Can you work these out from the model? Positions are in its coordinate system, mm. A direction names the side the tool comes from. Coordinates: 2 decimals unless noted, no trailing zeros. Order: outer loops, then holes, each group sorted by start corner. A loop starts at its lowest first (then second) coordinate and runs counter-clockwise, first axis right, second up. Notation, with made-up numbers: M -38,-1.5 L -22,-1.5 A12 ccw -22,3.5 Z; hole C 39.25,-3.75 d8. An arc over 180 degrees is marked long. Answer as a JSON object with one key per item and string values.
from build123d import *

# Parameters (mm, degrees)
F0_R     = 17.5
F1_DEPTH = 15
F2_R     = 2


with BuildPart() as f1:
    # F0 (on Top) → F1 (new body)
    with BuildSketch(Plane.XY):
        with BuildLine():
            Line((78.938091, 17.894301), (-76.061909, 17.894301))
            Line((-76.061909, 17.894301), (-76.061909, -7.105699))
            Line((-76.061909, -7.105699), (-76.061909, -37.105699))
            Line((-76.061909, -37.105699), (-66.061909, -37.105699))
            Line((-66.061909, -37.105699), (-66.061909, -7.105699))
            Line((-66.061909, -7.105699), (-58.411911, -7.105699))
            Line((-58.411911, -7.105699), (-51.411911, -21.471429))
            Line((-51.411911, -21.471429), (-44.411911, -7.105699))
            Line((-44.411911, -7.105699), (-31.055583, -7.105699))
            Line((-31.055583, -7.105699), (-31.055583, -22.105699))
            Line((-31.055583, -22.105699), (-23.055583, -22.105699))
            Line((-23.055583, -22.105699), (-23.055583, -7.105699))
            Line((-23.055583, -7.105699), (78.938091, -7.105699))
            ThreePointArc((78.938091, -7.105699), (146.629833, 5.394301), (78.938091, 17.894301))
        make_face()
        with Locations((111.629833, 5.394301)):
            Circle(F0_R, mode=Mode.SUBTRACT)
    extrude(amount=F1_DEPTH)

    # F2
    f2_edges = [f1.edges().sort_by_distance(p)[0] for p in [
        (1.438091, 17.894301, 15),
        (-76.061909, -9.605699, 15),
        (-71.061909, -37.105699, 15),
        (-66.061909, -22.105699, 15),
        (-62.23691, -7.105699, 15),
        (-54.911911, -14.288564, 15),
        (-47.911911, -14.288564, 15),
        (-37.733747, -7.105699, 15),
        (-31.055583, -14.605699, 15),
        (-27.055583, -22.105699, 15),
        (-23.055583, -14.605699, 15),
        (27.941254, -7.105699, 15),
        (146.629833, 5.394301, 15),
        (94.129833, 5.394301, 15),
    ]]
    fillet(f2_edges, radius=F2_R)


solid = f1.part
Item 1: I want a section at B-B, the plane z = 7.5. Write out the boundary of the cut face in (x, y), plus the area to 3 significant figures.
Answers follow:
{"outline": "M -76.06,-37.11 L -66.06,-37.11 L -66.06,-7.11 L -58.41,-7.11 L -51.41,-21.47 L -44.41,-7.11 L -31.06,-7.11 L -31.06,-22.11 L -23.06,-22.11 L -23.06,-7.11 L 78.94,-7.11 A35 ccw long 78.94,17.89 L -76.06,17.89 Z; hole C 111.63,5.39 d35", "area": "7,240 mm^2"}
Item 2: If we mould it in two halves opening along X, with no side actions, what happens to faces 1 (the flat face through (-76.062, -9, 6)), 2 (the cylindrical face through (-54.62, -13.585, 14.399)), 3 (the flat face through (-71, -37.106, 6))? For each: pulls with the +X half, pulls with the -X half, needs draft (parallel to the pull), parting line crosses it, or undercut.
Answers follow:
{"face 1": "pulls with the -X half", "face 2": "undercut", "face 3": "needs draft"}
Item 3: Which directions (+Z, -Z, +X, -X, +Y, -Y) give clear straight access to the entire face, cutting with the end or side of a thin tool? Please do faces 4 (the flat face through (3, 17.894, 6)), 5 (the flat face through (-23.056, -15, 6)), 6 (the cylindrical face through (-48.1, -13.37, 14.4)), 7 (the cylindrical face through (146.603, 4.034, 6.409)).
Answers follow:
{"face 4": "+Z, -Z, -X, +Y", "face 5": "+Z, -Z, -Y", "face 6": "+Z, -Y", "face 7": "+Z, -Z"}
Item 4: I'm going to push flat-ended pins straight in: pin 1 (5 mm diameter, centred on x = -20, z = 12, fed in from -Y); pin 2 (6 mm diameter, centred on y = -12.5, z = 4.5, fed in from +X); pin 3 (6.5 mm diameter, centred on y = -14, z = 8, fed in from +X). Where does each tip first touch, or does it pass through?
Answers follow:
{"pin 1": "stops at y = -7.11", "pin 2": "stops at x = 143.3", "pin 3": "stops at x = 142.68"}
Item 5: I want a section at A-A, the plane x = -35. Write out the boundary of the cut face in (y, z).
Answers follow:
{"outline": "M -7.11,0 L 17.89,0 L 17.89,13 A2 ccw 15.89,15 L -5.11,15 A2 ccw -7.11,13 Z"}
Item 6: Please list where these lines run through material, in increasing order: line 1 (X direction, y = -9.5, z = 4); line 2 (X direction, y = -22, z = 2.5); line 3 (Y direction, x = 50.5, z = 0.75).
Answers follow:
{"line 1": "x = -76.06 to -66.06, -57.25 to -45.58, -31.06 to -23.06, 79.96 to 102.44, 120.82 to 143.3", "line 2": "x = -76.06 to -66.06, -31.06 to -23.06, 89.85 to 133.41", "line 3": "y = -7.11 to 17.89"}
